Model file for the job. Use its own axes, mm. Face numbers are marked on the shaded views. Coordinates: 2 decimals unless noted, no trailing zeros. Loops run counter-clockwise (first coordinate to the right, second up) from the corner with the lowest first, then second, coordinate; pieces in that order, holes last.
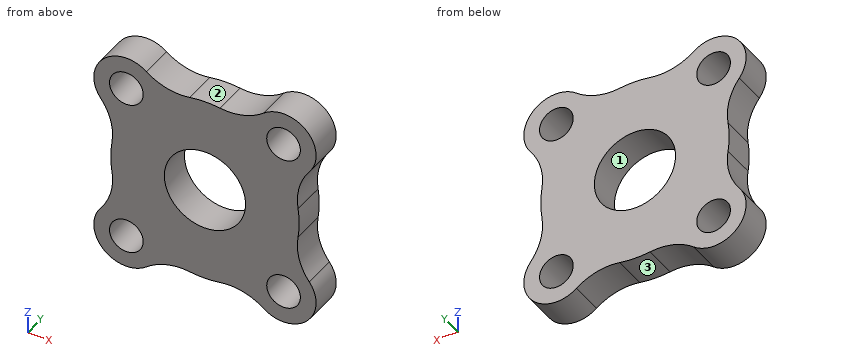
Autodesk Inventor part; units mm, degrees
ref_plane "YZ Plane" through (0, 0, 0) normal (1, 0, 0) x (0, 1, 0)
ref_plane "XZ Plane" through (0, 0, 0) normal (0, 1, 0) x (-1, 0, 0)
ref_plane "XY Plane" through (0, 0, 0) normal (0, 0, 1) x (1, 0, 0)
sketch "Эскиз1" plane through (0, 0, 0) normal (0, 1, 0) x (-1, 0, 0)
  circle A0 centre (0.1295, 0.2019) radius 7
  circle A1 centre (-6.8705, 7.2019) radius 1.5
  circle A2 centre (7.1295, 7.2019) radius 1.5
  circle A3 centre (7.1295, -6.7981) radius 1.5
  circle A4 centre (-6.8705, -6.7981) radius 1.5
  line L0 (-6.8705, -10.8093) -> (-6.8705, 13.8282) construction
  line L1 (14.3213, 7.2019) -> (-16.097, 7.2019) construction
  line L2 (7.1295, -11.068) -> (7.1295, 16.1729) construction
  arc A5 (6.5047, 14.6631) -> (7.1295, 16.1729) centre (4.9928, 16.1729) ccw construction
  line L3 (12.5583, -6.7981) -> (-15.6188, -6.7981) construction
  circle A6 centre (7.1295, 7.2019) radius 2.8995
  circle A7 centre (-6.8705, 7.2019) radius 2.8995
  circle A8 centre (-6.8705, -6.7981) radius 2.8995
  circle A9 centre (7.1295, -6.7981) radius 2.8995
  arc A10 (0.5599, -6.4772) -> (-0.2768, -6.4772) centre (0.1416, -8.4329) ccw
  line L4 (5.6295, -6.7981) -> (0.1295, -6.7981)
  line L5 (7.1295, -5.2981) -> (7.1295, 0.2019)
  line L6 (7.1295, 5.7019) -> (7.1295, 0.2019)
  line L7 (5.6295, 7.2019) -> (-5.3705, 7.2019)
  line L8 (-6.8705, 5.7019) -> (-6.8705, -5.2981)
  line L9 (-5.3705, -6.7981) -> (0.1295, -6.7981)
  circle A11 centre (0.1295, 0.2019) radius 8.3995
  circle A12 centre (0.1295, 0.2019) radius 3.6176
  point P0 (-3.971, 7.2019)
  point P1 (-6.8705, 4.3024)
  point P2 (-6.8705, -3.8986)
  point P3 (-3.971, -6.7981)
  point P4 (4.23, -6.7981)
  point P5 (7.1295, -3.8986)
  point P6 (7.1295, 4.3024)
  point P7 (4.23, 7.2019)
  point P8 (4.2478, 7.5225)
  point P9 (-3.9888, 7.5225)
  point P10 (-7.1911, 4.3202)
  point P11 (-7.1911, -3.9164)
  point P12 (-3.9888, -7.1187)
  point P13 (4.2478, -7.1187)
  point P14 (7.4501, -3.9164)
  point P15 (7.4501, 4.3202)
  dimension "d23" = 14
  dimension "d24" = 3
  dimension "d25" = 3
  dimension "d26" = 3
  dimension "d27" = 3
  dimension "d28" = 2
extrude "Выдавливание1" add sketch "Эскиз1" along normal blind 3 contours L5 A9 A0 | L6 A6 A11 A9 L5 | A0 A6 L6 | A0 L7 A6 | A6 L7 A11 L6 | A9 L4 A0 | A9 L5 A11 L4 | A9 A11 L5 | L6 A11 A6 | L7 A7 A11 A6 | A0 A7 L7 | A6 A11 L7 | L9 A8 A0 | L4 A9 A11 A8 L9 | L4 A11 A9 | A9 A11 L4 A3 L5 | L5 A3 A11 | A11 L6 A2 L7 A6 | A11 A2 L6 | A0 L8 A7 | A7 L8 A11 L7 | L7 A11 A7 | L7 A2 A11 | A8 L8 A0 | A8 L9 A11 L8 | A8 A11 L9 | A11 A3 L4 | L8 A8 A11 A7 | A7 A11 L8 | A11 L7 A1 L8 A7 | A11 A1 L7 | L8 A11 A8 | A8 A11 L8 A4 L9 | L9 A4 A11 | L8 A1 A11 | A11 A4 L8
extrude "Выдавливание3" add sketch "Эскиз1" along normal up to surface (3 mm away) contours A0
fillet "Сопряжение грани1" radius 5 2 edges at (-4.2478, 1.5, 7.5225) (-7.4501, 1.5, 4.3202)
fillet "Сопряжение грани2" radius 5 2 edges at (3.9888, 1.5, 7.5225) (7.1911, 1.5, 4.3202)
fillet_without_effect "Сопряжение грани3"
fillet "Сопряжение грани4" radius 5 2 edges at (7.1911, 1.5, -3.9164) (3.9888, 1.5, -7.1187)
fillet "Сопряжение грани5" radius 5 2 edges at (-4.2478, 1.5, -7.1187) (-7.4501, 1.5, -3.9164)
fillet_without_effect "Сопряжение грани6"
fillet_without_effect "Сопряжение грани7"
fillet_without_effect "Сопряжение грани8"
properties part number "крепление подшипника_1"
Q1. Slice it at D-D (y = 1.05). Count the separate pieces of the cut face and the enclosed holes in it, and give its area (3 significant figures).
Answers:
separate pieces: 1
enclosed holes: 5
area: 253 mm2
Q2. Slice it at B-B (z = 8). List the corners of the cut face in (x, y).
Answers:
outline: (-9.92, 0) - (-8.4, 0) - (-8.4, 3) - (-9.92, 3) - close; (-5.86, 0) - (5.6, 0) - (5.6, 3) - (-5.86, 3) - close; (8.14, 0) - (9.66, 0) - (9.66, 3) - (8.14, 3) - close
Q3. Flat gauge pins, fed straight in: P1, Ø4, axis at x = 6.87, z = 7.2, coming from the -Y side; P2, Ø1, axis at x = -0.5, y = 0.5, coming from the +Z side. Where does each tip first touch, or does it go through?
Answers:
P1: stops at y = 0
P2: stops at z = 8.6
Q4. Mould opens along Z. For the marked faces 1, 2 and 3 say: +Z half, -Z half, draft (parallel to the pull), parting line (faces both ways), or undercut.
Answers:
face 1: undercut
face 2: +Z half
face 3: -Z half
Q5. Drill centre lines: line 1 (X direction, y = 2.6, z = 6); line 2 (X direction, y = 0.65, z = 7.5); line 3 (Z direction, x = 1.5, y = 1.8). Where is each one in solid material? Low to high.
Answers:
line 1: x = -9.77 to -8.03, -6.23 to 5.97, 7.77 to 9.51
line 2: x = -10.01 to -8.6, -5.66 to 5.4, 8.34 to 9.75
line 3: z = -8.05 to -3.03, 3.43 to 8.46
Q6. Slice it at C-C (z = -0.25). List the corners of the cut face in (x, y), and give its area (3 significant figures).
Answers:
outline: (-8.52, 0) - (-3.72, 0) - (-3.72, 3) - (-8.52, 3) - close; (3.46, 0) - (8.26, 0) - (8.26, 3) - (3.46, 3) - close
area: 28.8 mm2
Q7. Slice it at A-A (x = 0). List the corners of the cut face in (y, z).
Answers:
outline: (0, -8.2) - (3, -8.2) - (3, -3.41) - (0, -3.41) - close; (0, 3.82) - (3, 3.82) - (3, 8.6) - (0, 8.6) - close
